```python
from build123d import *

# Parameters (mm, degrees)
F0_W     = 40
F0_H     = 40
F1_DEPTH = 40
F3_DEPTH = 10


with BuildPart() as f1:
    # F0 (on Front) → F1 (new body)
    with BuildSketch(Plane.XZ):
        Rectangle(F0_W, F0_H)
    extrude(amount=F1_DEPTH)

    # F2 (on Top) → F3 (join, symmetric)
    with BuildSketch(Plane.XY):
        Polygon((0, 0), (15, 0), (10, 20), (0, 20), align=None)
        Polygon((-15, 0), (0, 0), (0, 20), (-10, 20), align=None)
    extrude(amount=F3_DEPTH, both=True)


solid = f1.part
```
Geometry check sheet. Reference: the model listing, model coordinates, mm. A direction names the side the tool comes from. Coordinates: 2 decimals unless noted, no trailing zeros. Loops run counter-clockwise (first coordinate to the right, second up) from the corner with the lowest first, then second, coordinate; pieces in that order, holes last. Notation, with made-up numbers: (-8.75, 28.25) - (1.25, 28.25) arc R5 cw to (1.25, 34.25) - close; hole circle Ø11 at (-31.75, 16.5). An arc over 180 degrees is marked (long way). One line per item, written item: value. Start each with the question number.
(1) Cross-section at C-C on y = 10. Enter the section's corners in (x, z).
(2) Material ranges on line 1 (Y direction, x = -9.5, z = -15.5); line 2 (Z direction, x = 5, y = 5), recorded low to high. Write a range as [from, to].
(3) Depth check by flat-ended pin: P1, Ø1, axis at y = 8.5, z = -3, coming from the -X side; P2, Ø6, axis at x = 5.5, y = 10, coming from the -Z side; P3, Ø6, axis at x = 3, y = 8.5, coming from the +Z side. Enter the tip coordinate at first touch or a pass-through.
(4) Cross-section at D-D on z = 16. Enter the section's corners in (x, y), plus the area to 3 significant figures.
(5) Tool access check on faces 1 (the flat face through (20, -20, 0)), 2 (the flat face through (0, 10, 10)), 3 (the flat face through (0, 10, -10)). Record the directions out of +Z, -Z, +X, -X, +Y, -Y that give a thin tool (end or side, any length) a straight path to the whole face; none if there is none.
(6) Cross-section at B-B on x = -11. Enter the section's corners in (y, z).
(7) Cross-section at A-A on z = -7. Enter the section's corners in (x, y), plus the area to 3 significant figures.
Results below:
1. outline: (-12.5, -10) - (12.5, -10) - (12.5, 10) - (-12.5, 10) - close
2. line 1: y = [-40, 0]
2. line 2: z = [-10, 10]
3. P1: stops at x = -13
3. P2: stops at z = -10
3. P3: stops at z = 10
4. outline: (-20, -40) - (20, -40) - (20, 0) - (-20, 0) - close
4. area: 1,600 mm2
5. face 1: +Z, -Z, +X, +Y, -Y
5. face 2: +Z, +X, -X, +Y
5. face 3: -Z, +X, -X, +Y
6. outline: (-40, -20) - (0, -20) - (0, -10) - (16, -10) - (16, 10) - (0, 10) - (0, 20) - (-40, 20) - close
7. outline: (-20, -40) - (20, -40) - (20, 0) - (15, 0) - (10, 20) - (-10, 20) - (-15, 0) - (-20, 0) - close
7. area: 2,100 mm2
